Build history of the part. All positions in model axes, mm. Face numbers are marked on the shaded views. A direction names the side the tool comes from. Round coordinates to 2 decimals unless told otherwise and drop trailing zeros. Write each loop counter-clockwise with the first axis right and the second up, starting at its lowest first coordinate (ties: lowest second). Pieces come first, ordered by that corner, then holes. Notation, with made-up numbers: (-5.75, -18.5) -> (42.25, -18.5) arc R17 cw to (42.25, -3.5) -> close; hole circle Ø3 at (68, 22). An arc over 180 degrees is marked (long way). Return JSON: item names as keys, results as strings.
from build123d import *

# Parameters (mm, degrees)
F0_R      = 2
F1_DEPTH  = 5
F3_DEPTH  = 14.5
F4_R      = 2
F5_DEPTH  = 14.5
F7_DEPTH  = 25
F9_DEPTH  = 5
F11_DEPTH = 154
F12_R     = 2
F12_W     = 44.045060873
F12_H     = 72.3597388715
F13_DEPTH = 15
F15_DEPTH = 14.5
F16_R     = 2


with BuildPart() as f1:
    # F0 (on Top) → F1 (new body)
    with BuildSketch(Plane.XY):
        Polygon((-9, 9), (-9, -21), (21, 9), align=None)
        Circle(F0_R, mode=Mode.SUBTRACT)
    extrude(amount=F1_DEPTH)

    # F2 (on face) → F3 (join)
    with BuildSketch(Plane.XY.offset(5)):
        Polygon((-9, 9), (-9, -21), (-6.5, -18.5), (-6.5, 6.5), (18.5, 6.5), (21, 9), align=None)
    extrude(amount=F3_DEPTH)

    # F4 (on face) → F5 (cut, through all)
    with BuildSketch(Plane.XY.offset(19.5)):
        with Locations((-5.4393398282, 5.4393398282)):
            Circle(F4_R)
    extrude(amount=-F5_DEPTH, mode=Mode.SUBTRACT)

    # F6 (on face) → F7 (cut)
    with BuildSketch(Plane.XY.offset(19.5)):
        Polygon((18.5, 18.9713805318), (18.5, 6.5), (25.3656071275, -18.5), (25.3656071275, 18.9713805318), align=None)
        Polygon((-4.8339825459, -31.5633218139), (-6.5, -18.5), (-15.6000002623, -18.5), (-15.6000002623, -31.5633218139), align=None)
    extrude(amount=-F7_DEPTH, mode=Mode.SUBTRACT)

    # F8 (on face) → F9 (join, through all)
    with BuildSketch(Plane.XY.offset(5)):
        Polygon((18.5, -4), (18.5, 6.5), (8, -4), align=None)
    extrude(amount=-F9_DEPTH)

    # F10 (on face) → F11 (join)
    with BuildSketch(Plane.YZ.offset(18.5)):
        Polygon((-4, 5), (-4, 0), (9, 0), (9, 19.5), (6.5, 19.5), (6.5, 5), align=None)
    extrude(amount=F11_DEPTH)

    # F12 (on face) → F13 (cut, symmetric)
    with BuildSketch(Plane.XY.offset(5)):
        with Locations((145, 0)):
            Circle(F12_R)
        with Locations((170.5225304365, -14.2861837521)):
            Rectangle(F12_W, F12_H)
    extrude(amount=F13_DEPTH, both=True, mode=Mode.SUBTRACT)

    # F14 (on face) → F15 (join, through all)
    with BuildSketch(Plane.XY.offset(5)):
        with BuildLine():
            Line((15.2678268764, 6.5), (4.7321731236, 6.5))
            ThreePointArc((4.7321731236, 6.5), (10, 5), (15.2678268764, 6.5))
        make_face()
        with BuildLine():
            Line((-6.5, -4.7321731236), (-6.5, -15.2678268764))
            ThreePointArc((-6.5, -15.2678268764), (-5, -10), (-6.5, -4.7321731236))
        make_face()
    extrude(amount=F15_DEPTH)

    # F16
    f16_edges = [f1.edges().sort_by_distance(p)[0] for p in [
        (148.5, 6.5, 12.25),
    ]]
    fillet(f16_edges, radius=F16_R)


with BuildPart() as f17_1:
    # F17: instance of F1
    add(f1.part.mirror(Plane(origin=(69.75, 9, 9.75), x_dir=(-1, 0, 0), z_dir=(0, 1, 0))))


solid = f17_1.part
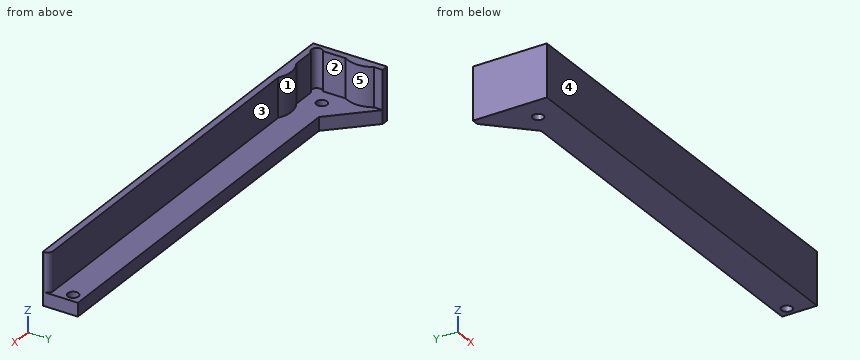
Q1. Wall check: L1, parallel to X at y = 18, z = 2.5; L2, parallel to Y at x = 145, z = 3.7; L3, parallel to Y at x = 22.5, z = 8.5. Give the ranges that are in metal, low to high.
Verdict:
{"L1": "x = -9 to -2, 2 to 143, 147 to 148.5", "L2": "y = 9 to 16, 20 to 22", "L3": "y = 9 to 11.5"}
Q2. Saw through at D-D on x = 47. List the corners of the cut face in (y, z).
Verdict:
{"outline": "(9, 0) -> (22, 0) -> (22, 5) -> (11.5, 5) -> (11.5, 19.5) -> (9, 19.5) -> close"}
Q3. Pin check, flat tips, straight feed: pin 1 Ø1.5 at (y, z) = (16, 14) entering from +X; pin 2 Ø4 at (x, z) = (91.5, 2.5) entering from +Y; pin 3 Ø3.5 at (y, z) = (34.5, 12) entering from +X. Stop position of each tip, or through.
Verdict:
{"pin 1": "stops at x = -6.5", "pin 2": "stops at y = 22", "pin 3": "stops at x = -6.2"}
Q4. Two-plate mould, pull along X, no slides. Class the marked faces 1, 2 and 3: +X half, -X half, draft (parallel to the pull), parting line (faces both ways), or undercut.
Verdict:
{"face 1": "undercut", "face 2": "+X half", "face 3": "draft"}
Q5. Saw through at B-B on y = 18. List the corners of the cut face in (x, z).
Verdict:
{"outline": "(-9, 0) -> (-2, 0) -> (-2, 5) -> (-6.5, 5) -> (-6.5, 19.5) -> (-9, 19.5) -> close; (2, 0) -> (143, 0) -> (143, 5) -> (2, 5) -> close; (147, 0) -> (148.5, 0) -> (148.5, 5) -> (147, 5) -> close"}
Q6. Saw through at C-C on z = 16.5. List the corners of the cut face in (x, y), then the cut area to 3 significant figures.
Verdict:
{"outline": "(-9, 9) -> (148.5, 9) -> (148.5, 9.5) arc R2 ccw to (146.5, 11.5) -> (15.27, 11.5) arc R10 ccw to (4.73, 11.5) -> (-3.74, 11.5) arc R2 cw (long way) to (-6.5, 14.26) -> (-6.5, 22.73) arc R10 ccw to (-6.5, 33.27) -> (-6.5, 36.5) -> (-9, 36.5) -> close", "area": "473 mm²"}
Q7. Saw through at A-A on x = 0. List the corners of the cut face in (y, z), then the cut area to 3 significant figures.
Verdict:
{"outline": "(9, 0) -> (16, 0) -> (16, 5) -> (11.5, 5) -> (11.5, 19.5) -> (9, 19.5) -> close; (20, 0) -> (30, 0) -> (30, 5) -> (20, 5) -> close", "area": "121 mm²"}
Q8. 3-axis set-ups, long thin cutter, end or side, ignore diameter. For the marked faces 4 and 5: which of +Z, -Z, +X, -X, +Y, -Y reach the whole face in a straight line?
Verdict:
{"face 4": "+Z, -Z, +X, -X, -Y", "face 5": "+Z, +X"}
